Autodesk Inventor part; units mm, degrees
ref_plane "YZ Plane" through (0, 0, 0) normal (1, 0, 0) x (0, 1, 0)
ref_plane "XZ Plane" through (0, 0, 0) normal (0, 1, 0) x (-1, 0, 0)
ref_plane "XY Plane" through (0, 0, 0) normal (0, 0, 1) x (1, 0, 0)
sketch "Sketch1" plane through (0, 0, 0) normal (1, 0, 0) x (0, 1, 0)
  arc A0 (31, -20.1145) -> (-31, -42) centre (65.6672, -217.087) ccw
  line L0 (-31, 42) -> (31, 42) construction
  line L1 (31, 42) -> (31, -42) construction
  line L2 (31, -42) -> (-31, -42) construction
  line L3 (-31, -42) -> (-31, 42)
  line L4 (31, 0) -> (-31, 0) construction
  arc A1 (-31, 42) -> (31, 20.1145) centre (65.6672, 217.087) ccw
  line L5 (31, 20.1145) -> (31, -20.1145)
  point P0 (0, 0)
  point P1 (0, 42)
  dimension "d0" = 400
  dimension "d1" = 62
  dimension "d2" = 84
  dimension "d23" = 40.2289
extrude "Extrusion1" add sketch "Sketch1" along normal mid plane 14
sketch "Sketch2" plane through (7, 0, 0) normal (1, 0, 0) x (0, 0, -1)
  arc A0 (-42, -31) -> (-20.1145, 31) centre (-217.087, 65.6672) ccw construction
  line L0 (-42, -31) -> (42, -31) construction
  arc A1 (20.1145, 31) -> (42, -31) centre (217.087, 65.6672) ccw construction
  line L1 (20.1145, 31) -> (-20.1145, 31) construction
  line L2 (-16.6, -12.2) -> (-8.4, -12.2)
  line L3 (-8.4, -12.2) -> (-8.4, -15)
  line L4 (-8.4, -15) -> (-16.6, -15)
  line L5 (-16.6, -15) -> (-16.6, -12.2)
  line L6 (0, 0) -> (0, -31) construction
  line L7 (-42, -31) -> (42, -31) construction
  line L8 (16.6, -12.2) -> (8.4, -12.2)
  line L9 (8.4, -12.2) -> (8.4, -15)
  line L10 (8.4, -15) -> (16.6, -15)
  line L11 (16.6, -15) -> (16.6, -12.2)
  line L12 (-4.1, 23.8) -> (4.1, 23.8)
  line L13 (4.1, 23.8) -> (4.1, 21)
  line L14 (4.1, 21) -> (-4.1, 21)
  line L15 (-4.1, 21) -> (-4.1, 23.8)
  point P0 (12.5, -12.2)
  point P1 (-12.5, -12.2)
  point P2 (0, 23.8)
  dimension "d6" = 8.2
  dimension "d7" = 2.8
  dimension "d8" = 16
  dimension "d9" = 25
  dimension "d16" = 8.2
  dimension "d17" = 2.8
  dimension "d19" = 10
extrude "Extrusion2" cut sketch "Sketch2" against normal through all
sketch "Sketch3" plane through (-7, -31, -42) normal (0, -1, 0) x (1, 0, 0)
  line L0 (0, 0) -> (14, 0) construction
  line L1 (14, 84) -> (14, 0) construction
  line L2 (0, 84) -> (14, 84) construction
  line L3 (0, 0) -> (0, 84) construction
  line L4 (14, 42) -> (0, 42) construction
  line L5 (0, 0) -> (0, 84) construction
  line L6 (0, 84) -> (14, 84) construction
  line L7 (7, 84) -> (7, 0) construction
  line L8 (0, 0) -> (14, 0) construction
  circle A0 centre (7, 54.5) radius 2.75
  circle A1 centre (7, 29.5) radius 2.75
  point P0 (7, 42)
  dimension "d12" = 5.5
  dimension "d13" = 25
extrude "Extrusion3" cut sketch "Sketch3" against normal blind 25
sketch "Sketch4" plane through (-7, 31, 20.1145) normal (0, 1, 0) x (1, 0, 0)
  line L0 (14, 0) -> (0, 0) construction
  line L1 (14, 40.2289) -> (14, 0) construction
  line L2 (0, 40.2289) -> (14, 40.2289) construction
  line L3 (0, 0) -> (0, 40.2289) construction
  line L4 (0, 20.1145) -> (14, 20.1145) construction
  line L5 (14, 16.0145) -> (14, 24.2145) construction
  line L6 (14, 0) -> (0, 0) construction
  line L7 (7, 0) -> (7, 40.2289) construction
  line L8 (0, 40.2289) -> (14, 40.2289) construction
  circle A0 centre (7, 20.1145) radius 2.75
  dimension "d20" = 5.5
extrude "Extrusion4" cut sketch "Sketch4" against normal blind 15
properties part number "cuerpo_obj1"
Geometry: final body of the model. Coordinates: model frame, mm. A direction names the side the tool comes from. Give positions to 0.01 mm unless a question says otherwise; leave off trailing zeros. Order: outer loops, then holes, each group sorted by start corner. A loop starts at its lowest first (then second) coordinate and runs counter-clockwise, first axis right, second up. Notation, with made-up numbers: (80, 18.5) -> (115, 18.5) arc R17 ccw to (115, 37.5) -> close; hole circle Ø5 at (-30.5, -14.75). An arc over 180 degrees is marked (long way). Answer as a JSON object with one key per item and string values.
Q1. Material intervals for probe 1 along Y at (x, z) = (4, 1); probe 2 along Y at (x, z) = (4.5, 13); probe 3 along Z at (x, y) = (0, -10.5), sorted ascending.
Entries:
{"probe 1": "y = -31 to 21, 23.8 to 31", "probe 2": "y = -31 to -15, -12.2 to 31", "probe 3": "z = -32.16 to -15.25, -9.75 to 9.75, 15.25 to 32.16"}
Q2. Draft query along Y for faces 6 (the flat face through (0, 23.8, 3)), 7 (the flat face through (0, -6, -12)), 8 (the flat face through (-3, 31, 0)), 9 (the cylindrical face through (-2.027, -9.143, 14.359)). Return one class per face: released by +Y, released by -Y, zero draft, split by the parting line, or undercut.
Entries:
{"face 6": "undercut", "face 7": "released by -Y", "face 8": "released by +Y", "face 9": "zero draft"}
Q3. Section A-A (z = 0). Output: boundary loops of the cut face in (x, y).
Entries:
{"outline": "(-7, -31) -> (7, -31) -> (7, 21) -> (2.75, 21) -> (2.75, 16) -> (-2.75, 16) -> (-2.75, 21) -> (-7, 21) -> close; (-7, 23.8) -> (-2.75, 23.8) -> (-2.75, 31) -> (-7, 31) -> close; (2.75, 23.8) -> (7, 23.8) -> (7, 31) -> (2.75, 31) -> close"}
Q4. Section B-B (x = -5.75). Output: boundary loops of the cut face in (y, z).
Entries:
{"outline": "(-31, -42) arc R200 cw to (31, -20.11) -> (31, 20.11) arc R200 cw to (-31, 42) -> close; hole (-15, -16.6) -> (-12.2, -16.6) -> (-12.2, -8.4) -> (-15, -8.4) -> close; hole (-15, 8.4) -> (-12.2, 8.4) -> (-12.2, 16.6) -> (-15, 16.6) -> close; hole (21, -4.1) -> (23.8, -4.1) -> (23.8, 4.1) -> (21, 4.1) -> close"}
Q5. First-contact query: pin 1 (5 mm diameter, centred on x = 1, y = 12.5, fed in from -Z); pin 2 (3 mm diameter, centred on x = -0.5, y = -14, fed in from -Z); pin 3 (8 mm diameter, centred on x = -5, y = -11.5, fed in from +Z). Flat tips, straight axial feed; report the tip coordinate or a pass-through.
Entries:
{"pin 1": "stops at z = -24.99", "pin 2": "stops at z = -34.3", "pin 3": "stops at z = 34.3"}
Q6. Section C-C (y = -7). Output: boundary loops of the cut face in (x, z).
Entries:
{"outline": "(-7, -30.76) -> (7, -30.76) -> (7, 30.76) -> (-7, 30.76) -> close; hole circle Ø5.5 at (0, -12.5); hole circle Ø5.5 at (0, 12.5)"}
Q7. Section D-D (z = 12.5). Output: boundary loops of the cut face in (x, y).
Entries:
{"outline": "(-7, -31) -> (-2.75, -31) -> (-2.75, -15) -> (-7, -15) -> close; (-7, -12.2) -> (-2.75, -12.2) -> (-2.75, -6) -> (2.75, -6) -> (2.75, -12.2) -> (7, -12.2) -> (7, 31) -> (-7, 31) -> close; (2.75, -31) -> (7, -31) -> (7, -15) -> (2.75, -15) -> close"}
Q8. Access query for faces 1 (the flat face through (0, -6, 13)), 2 (the cylindrical face through (-0.596, 18.535, 2.685)), 3 (the flat face through (0, 22, -4.1)), 4 (the flat face through (-7, 0, 1)), 5 (the cylindrical face through (-0.1, -0.47, 28.34)). Directions: +Z, -Z, +X, -X, +Y, -Y. A direction counts if a zero-diameter tool reaches every point of the face in a straight line with its end or side. Return the directions, or none.
Entries:
{"face 1": "-Y", "face 2": "+Y", "face 3": "+X, -X", "face 4": "+Z, -Z, -X, +Y, -Y", "face 5": "+Z, +X, -X, +Y"}
